Part model, mm, in its own coordinate system. A direction names the side the tool comes from. Round coordinates to 2 decimals unless told otherwise and drop trailing zeros. Loops run counter-clockwise (first coordinate to the right, second up) from the corner with the lowest first, then second, coordinate; pieces in that order, holes last.
(1) Tool access for faces 1 (the face through (36, 0, 21.59)), 2 (the face through (-31.877, -19, 10)), 3 (the face through (14.476, -30.14, 20.866)): list every direction of +Z, -Z, +X, -X, +Y, -Y with a clear straight run to the whole face (end or side of a thin tool).
(2) Mould opens along Y. For faces 4 (the face through (-15.24, 30, 9)), 5 (the face through (-1, -31.75, 24)), 6 (the face through (36, 9.525, 9)), 7 (the face through (-34.544, -23.55, 12.878)) say: +Y half, -Y half, draft (parallel to the pull), parting line (faces both ways), or undercut.
(3) Cut at A-A on z = 5.5. Count the separate pieces of the cut face and the enclosed holes in it, then the cut area to 3 significant figures.
(4) Flat gauge pins, fed straight in: pin 1 (2.5 mm diameter, centred on x = -35.5, y = -2, fed in from -Z); pin 2 (1.6 mm diameter, centred on y = 30.5, z = 7.5, fed in from +X); pin 3 (3 mm diameter, centred on x = -25.5, y = -7, fed in from -Z); pin 4 (7 mm diameter, centred on x = 11.5, z = 16.5, fed in from -Y). Where does each tip first touch, or does it go through?
(5) Cut at C-C on y = 1.5. List the corners of the cut face in (x, z) (3 decimals).
(6) Cut at B-B on x = -7. List the corners of the cut face in (y, z) (3 decimals), then the cut area to 3 significant figures.
(7) Cut at D-D on y = -24.13. List the corners of the cut face in (x, z) (3 decimals), then the cut area to 3 significant figures.
(8) Probe probe 1 along X at (y, z) = (12, 6.5) (3 decimals); probe 2 along Y at (x, z) = (-17, 7.75) (3 decimals); probe 3 along Y at (x, z) = (32.5, 4) (3 decimals). List the from-to ranges inside material, lowest first.
from build123d import *

# Parameters (mm, degrees)
SKETCH1_W             = 80.01
SKETCH1_H             = 63.5
BOSS_EXTRUDE1_DEPTH   = 25.4
SKETCH2_W             = 63.754
SKETCH2_H             = 57.15
CUT_EXTRUDE1_DEPTH    = 22.86
F_8_CLEARANCE_HOLE1_D = 3.8608
SKETCH13_W            = 20.32
SKETCH13_H            = 21.59
CUT_EXTRUDE3_DEPTH    = 50.8
SKETCH14_W            = 8.128
SKETCH14_H            = 19.05
CUT_EXTRUDE4_DEPTH    = 21.59
SKETCH15_W            = 30.48
SKETCH15_H            = 3.175
CUT_EXTRUDE5_DEPTH    = 21.59
FILLET1_R             = 2.54
FILLET2_R             = 2.54
FILLET3_R             = 2.54


with BuildPart() as part:
    # Sketch1 → Boss-Extrude1 (new body)
    with BuildSketch(Plane.XY):
        Rectangle(SKETCH1_W, SKETCH1_H)
    extrude(amount=BOSS_EXTRUDE1_DEPTH)

    # Sketch2 → Cut-Extrude1 (cut)
    with BuildSketch(Plane.XY):
        Rectangle(SKETCH2_W, SKETCH2_H)
    extrude(amount=CUT_EXTRUDE1_DEPTH, mode=Mode.SUBTRACT)

    # #8 Clearance Hole1 (through all)
    with Locations(Plane(origin=(0, 0, 0), x_dir=(-1, 0, 0), z_dir=(0, 0, -1))):
        with Locations((-36.3855, -24.13), (-36.3855, 24.13), (36.3855, 24.13), (36.3855, -24.13)):
            Hole(F_8_CLEARANCE_HOLE1_D / 2)

    # Sketch13 → Cut-Extrude3 (cut)
    with BuildSketch(Plane(origin=(0, 0, 0), x_dir=(1, 0, 0), z_dir=(0, 1, 0))):
        with Locations((0, -10.795)):
            Rectangle(SKETCH13_W, SKETCH13_H)
    extrude(amount=-CUT_EXTRUDE3_DEPTH, mode=Mode.SUBTRACT)

    # Sketch14 → Cut-Extrude4 (cut)
    with BuildSketch(Plane(origin=(0, 0, 0), x_dir=(-1, 0, 0), z_dir=(0, 0, -1))):
        with Locations((-35.941, 0)):
            Rectangle(SKETCH14_W, SKETCH14_H)
        with Locations((35.941, 0)):
            Rectangle(SKETCH14_W, SKETCH14_H)
    extrude(amount=-CUT_EXTRUDE4_DEPTH, mode=Mode.SUBTRACT)

    # Sketch15 → Cut-Extrude5 (cut)
    with BuildSketch(Plane(origin=(0, 0, 0), x_dir=(-1, 0, 0), z_dir=(0, 0, -1))):
        with Locations((0, 30.1625)):
            Rectangle(SKETCH15_W, SKETCH15_H)
        with Locations((0, -30.1625)):
            Rectangle(SKETCH15_W, SKETCH15_H)
    extrude(amount=-CUT_EXTRUDE5_DEPTH, mode=Mode.SUBTRACT)

    # Fillet1
    # the kernel refuses this fillet: 2.54 mm, written as the material it adds along each edge
    with BuildSketch(Plane(origin=(31.877, -28.575, 22.86), x_dir=(0, 0, -1), z_dir=(0, 1, 0))) as fillet1_piece_1_section:
        with BuildLine():
            CenterArc((FILLET1_R, FILLET1_R), FILLET1_R, 180, 90)
            Line((0, FILLET1_R), (0, 0))
            Line((0, 0), (FILLET1_R, 0))
        make_face()
    fillet1_piece_1 = extrude(amount=63.5, mode=Mode.PRIVATE)
    fillet1_piece_1 = split(fillet1_piece_1, bisect_by=Plane(origin=(31.776201135, -9.525, 21.276910424), z_dir=(0, -1, 0)), keep=Keep.TOP, mode=Mode.PRIVATE)
    add(fillet1_piece_1)
    with BuildSketch(Plane(origin=(31.877, -34.925, 22.86), x_dir=(0, 0, -1), z_dir=(0, 1, 0))) as fillet1_piece_2_section:
        with BuildLine():
            CenterArc((FILLET1_R, FILLET1_R), FILLET1_R, 180, 90)
            Line((0, FILLET1_R), (0, 0))
            Line((0, 0), (FILLET1_R, 0))
        make_face()
    fillet1_piece_2 = extrude(amount=63.5, mode=Mode.PRIVATE)
    fillet1_piece_2 = split(fillet1_piece_2, bisect_by=Plane(origin=(31.257176883, 0, 21.59), z_dir=(0, 0, 1)), keep=Keep.TOP, mode=Mode.PRIVATE)
    fillet1_piece_2 = split(fillet1_piece_2, bisect_by=Plane(origin=(31.257176883, -9.525, 22.406874338), z_dir=(0, 1, 0)), keep=Keep.TOP, mode=Mode.PRIVATE)
    add(fillet1_piece_2)
    with BuildSketch(Plane(origin=(31.877, -34.925, 22.86), x_dir=(0, 0, -1), z_dir=(0, 1, 0))) as fillet1_piece_3_section:
        with BuildLine():
            CenterArc((FILLET1_R, FILLET1_R), FILLET1_R, 180, 90)
            Line((0, FILLET1_R), (0, 0))
            Line((0, 0), (FILLET1_R, 0))
        make_face()
    fillet1_piece_3 = extrude(amount=63.5, mode=Mode.PRIVATE)
    fillet1_piece_3 = split(fillet1_piece_3, bisect_by=Plane(origin=(31.776201135, 9.525, 21.276910424), z_dir=(0, 1, 0)), keep=Keep.TOP, mode=Mode.PRIVATE)
    add(fillet1_piece_3)
    with BuildSketch(Plane(origin=(-31.877, 28.575, 22.86), x_dir=(1, 0, 0), z_dir=(0, -1, 0))) as fillet1_piece_4_section:
        with BuildLine():
            CenterArc((FILLET1_R, -FILLET1_R), FILLET1_R, 90, 90)
            Line((0, -FILLET1_R), (0, 0))
            Line((0, 0), (FILLET1_R, 0))
        make_face()
    fillet1_piece_4 = extrude(amount=57.15, mode=Mode.PRIVATE)
    fillet1_piece_4 = split(fillet1_piece_4, bisect_by=Plane(origin=(-31.257176883, 19.05, 21.59), z_dir=(0, 0, 1)), keep=Keep.TOP, mode=Mode.PRIVATE)
    add(fillet1_piece_4)
    with BuildSketch(Plane(origin=(-31.877, 28.575, 22.86), x_dir=(1, 0, 0), z_dir=(0, -1, 0))) as fillet1_piece_5_section:
        with BuildLine():
            CenterArc((FILLET1_R, -FILLET1_R), FILLET1_R, 90, 90)
            Line((0, -FILLET1_R), (0, 0))
            Line((0, 0), (FILLET1_R, 0))
        make_face()
    fillet1_piece_5 = extrude(amount=63.5, mode=Mode.PRIVATE)
    fillet1_piece_5 = split(fillet1_piece_5, bisect_by=Plane(origin=(-31.776201135, 9.525, 21.276910424), z_dir=(0, 1, 0)), keep=Keep.TOP, mode=Mode.PRIVATE)
    add(fillet1_piece_5)
    with BuildSketch(Plane(origin=(-31.877, 34.925, 22.86), x_dir=(1, 0, 0), z_dir=(0, -1, 0))) as fillet1_piece_6_section:
        with BuildLine():
            CenterArc((FILLET1_R, -FILLET1_R), FILLET1_R, 90, 90)
            Line((0, -FILLET1_R), (0, 0))
            Line((0, 0), (FILLET1_R, 0))
        make_face()
    fillet1_piece_6 = extrude(amount=63.5, mode=Mode.PRIVATE)
    fillet1_piece_6 = split(fillet1_piece_6, bisect_by=Plane(origin=(-31.776201135, -9.525, 21.276910424), z_dir=(0, -1, 0)), keep=Keep.TOP, mode=Mode.PRIVATE)
    add(fillet1_piece_6)

    # Fillet2
    fillet2_edges = [part.edges().sort_by_distance(p)[0] for p in [
        (-15.24, 30.1625, 21.59),
        (15.24, 30.1625, 21.59),
        (15.24, -30.1625, 21.59),
        (-15.24, -30.1625, 21.59),
        (-35.770852263, 9.525, 21.59),
        (-35.770852263, -9.525, 21.59),
        (35.770852263, -9.525, 21.59),
        (35.770852263, 9.525, 21.59),
    ]]
    fillet(fillet2_edges, radius=FILLET2_R)

    # Fillet3
    fillet3_edges = [part.edges().sort_by_distance(p)[0] for p in [
        (-40.005, 31.75, 12.7),
        (40.005, 31.75, 12.7),
        (40.005, -31.75, 12.7),
        (-40.005, -31.75, 12.7),
    ]]
    fillet(fillet3_edges, radius=FILLET3_R)


solid = part.part
Final values:
1. face 1: -Z, +X, -X
1. face 2: -Z
1. face 3: -Z, +Y, -Y
2. face 4: draft
2. face 5: -Y half
2. face 6: undercut
2. face 7: undercut
3. separate pieces: 4
3. enclosed holes: 4
3. area: 882 mm2
4. pin 1: stops at z = 21.59
4. pin 2: stops at x = 39.96
4. pin 3: stops at z = 22.86
4. pin 4: passes through
5. outline: (-40.005, 21.59) - (-31.537, 21.59) arc R2.54 cw to (-29.337, 22.86) - (29.337, 22.86) arc R2.54 cw to (31.537, 21.59) - (40.005, 21.59) - (40.005, 25.4) - (-40.005, 25.4) - close
6. outline: (-31.75, 21.59) - (-28.575, 21.59) - (-28.575, 22.86) - (28.575, 22.86) - (28.575, 21.59) - (31.75, 21.59) - (31.75, 25.4) - (-31.75, 25.4) - close
6. area: 169 mm2
7. outline: (-40.005, 0) - (-38.316, 0) - (-38.316, 25.4) - (-40.005, 25.4) - close; (-34.455, 0) - (-31.877, 0) - (-31.877, 20.32) arc R2.54 cw to (-29.337, 22.86) - (29.337, 22.86) arc R2.54 cw to (31.877, 20.32) - (31.877, 0) - (34.455, 0) - (34.455, 25.4) - (-34.455, 25.4) - close; (38.316, 0) - (40.005, 0) - (40.005, 25.4) - (38.316, 25.4) - close
7. area: 381 mm2
8. probe 1: x = -40.005 to -31.877, 31.877 to 40.005
8. probe 2: y = -31.75 to -28.575, 28.575 to 31.75
8. probe 3: y = -31.75 to -9.525, 9.525 to 31.75
